Could you check a few things on this model? Use its own coordinates, in mm. A direction names the side the tool comes from. Coordinates: 2 decimals unless noted, no trailing zeros. Write each loop counter-clockwise with the first axis right and the second up, starting at its lowest first coordinate (ties: lowest second). Pieces come first, ordered by that corner, then holes.
Item 1: If I drill on probe 1 along Z at (x, y) = (192, 73); probe 2 along Z at (x, y) = (192.5, 71.75); probe 3 along Z at (x, y) = (112, 81.5), over which ranges is the centre line in solid material (lowest first)?
Item 2: I want a section at B-B on y = 46. Please give me the cut outline in (x, z).
Item 3: I want a section at A-A on x = 130. Please give me the cut outline in (y, z).
Item 4: I want a section at D-D on x = 38. Please give me the cut outline in (y, z).
Item 5: I want a section at C-C on z = 22.5. Please give me the cut outline in (x, y).
Item 6: For P1, Ø2, axis at x = 125, z = 103.5, coming from the +Y side; P2, Ø10, axis at x = 205.5, z = 72.5, coming from the -Y side; P3, Ø11, axis at y = 73.5, z = 60, coming from the +X side, each with a flat end and sliding along its axis, tell me the tip position at first contact or that it passes through.
Item 7: Which directions (+Z, -Z, +X, -X, +Y, -Y) give clear straight access to the entire face, cutting with the end or side of a thin tool? Please do faces 1 (the flat face through (77.5, 75, 64)), 2 (the cylindrical face through (219.827, 57.621, 42.078)), 3 (the cylindrical face through (80.452, 57.023, 42.078)), 4 (the flat face through (222.5, 75, 64)).
from build123d import *

# Parameters (mm, degrees)
SKETCH1_W                       = 300
SKETCH1_H                       = 150
BOSS_EXTRUDE1_DEPTH             = 15
BOSS_EXTRUDE2_DEPTH             = 100
CUT_EXTRUDE1_DEPTH              = 301
F_5_0_2055_DIAMETER_HOLE1_D     = 5.2197
F_5_0_2055_DIAMETER_HOLE1_DEPTH = 25
F_5_0_2055_DIAMETER_HOLE1_TIP   = 1.568156087


with BuildPart() as part:
    # Sketch1 → Boss-Extrude1 (new body)
    with BuildSketch(Plane.XY):
        with Locations((150, 75)):
            Rectangle(SKETCH1_W, SKETCH1_H)
    extrude(amount=BOSS_EXTRUDE1_DEPTH)

    # Sketch2 → Boss-Extrude2 (add)
    with BuildSketch(Plane.XY.offset(15)):
        with BuildLine():
            Line((77.5, 80), (222.5, 80))
            Line((222.5, 80), (222.5, 70))
            ThreePointArc((222.5, 70), (213.713203436, 48.786796564), (192.5, 40))
            Line((192.5, 40), (107.5, 40))
            ThreePointArc((107.5, 40), (86.286796564, 48.786796564), (77.5, 70))
            Line((77.5, 70), (77.5, 80))
        make_face()
    extrude(amount=BOSS_EXTRUDE2_DEPTH)

    # Sketch3 → Cut-Extrude1 (cut, through all)
    with BuildSketch(Plane(origin=(0, 0, 0), x_dir=(0, 0, -1), z_dir=(1, 0, 0))):
        Polygon((-115, 70), (-15, 40), (-115, 40), align=None)
    extrude(amount=CUT_EXTRUDE1_DEPTH, mode=Mode.SUBTRACT)

    # #5 (0.2055) Diameter Hole1
    with Locations(Plane(origin=(0, 80, 0), x_dir=(1, 0, 0), z_dir=(0, 1, 0))):
        with Locations((107.5, -86.041301647), (192.5, -86.041301647)):
            Hole(F_5_0_2055_DIAMETER_HOLE1_D / 2, depth=F_5_0_2055_DIAMETER_HOLE1_DEPTH)
            with Locations((0, 0, -(F_5_0_2055_DIAMETER_HOLE1_DEPTH + F_5_0_2055_DIAMETER_HOLE1_TIP / 2))):  # 118° drill point
                Cone(0, F_5_0_2055_DIAMETER_HOLE1_D / 2, F_5_0_2055_DIAMETER_HOLE1_TIP, mode=Mode.SUBTRACT)


solid = part.part
Response values:
1. probe 1: z = 0 to 83.48, 88.6 to 115
1. probe 2: z = 0 to 83.43, 88.65 to 115
1. probe 3: z = 0 to 15
2. outline: (0, 0) - (300, 0) - (300, 15) - (210.5, 15) - (210.5, 35) - (89.5, 35) - (89.5, 15) - (0, 15) - close
3. outline: (0, 0) - (150, 0) - (150, 15) - (80, 15) - (80, 115) - (70, 115) - (40, 15) - (0, 15) - close
4. outline: (0, 0) - (150, 0) - (150, 15) - (0, 15) - close
5. outline: (77.5, 70) arc R30 ccw to (96.1, 42.25) - (203.9, 42.25) arc R30 ccw to (222.5, 70) - (222.5, 80) - (77.5, 80) - close
6. P1: stops at y = 80
6. P2: stops at y = 55.75
6. P3: stops at x = 222.5
7. face 1: +Z, -X, +Y, -Y
7. face 2: +Z, +X, -Y
7. face 3: +Z, -X, -Y
7. face 4: +Z, +X, +Y, -Y
